```python
from build123d import *

# Parameters (mm, degrees)
F0_W     = 50.8
F0_H     = 50.8
F2_DEPTH = 50.8
F1_R     = 12.7
F3_DEPTH = 51.308
F4_W     = 25.4
F4_H     = 25.4
F5_DEPTH = 12.7
F6_R     = 14.097
F7_DEPTH = 12.7


with BuildPart() as f2:
    # F0 (on Front) → F2 (new body)
    with BuildSketch(Plane.XZ):
        with Locations((-25.4, 25.4)):
            Rectangle(F0_W, F0_H)
    extrude(amount=F2_DEPTH)

    # F1 (on face) → F3 (cut)
    with BuildSketch(Plane.XZ):
        with Locations((-25.4, 25.4)):
            Circle(F1_R)
    extrude(amount=F3_DEPTH, mode=Mode.SUBTRACT)

    # F4 (on face) → F5 (join)
    with BuildSketch(Plane.YZ):
        with Locations((-25.4, 25.4)):
            Rectangle(F4_W, F4_H)
    extrude(amount=F5_DEPTH)

    # F6 (on face) → F7 (join)
    with BuildSketch(Plane(origin=(0, 0, 0), x_dir=(1, 0, 0), z_dir=(0, 0, -1))):
        with Locations((-25.4, 25.4)):
            Circle(F6_R)
    extrude(amount=F7_DEPTH)


solid = f2.part
```
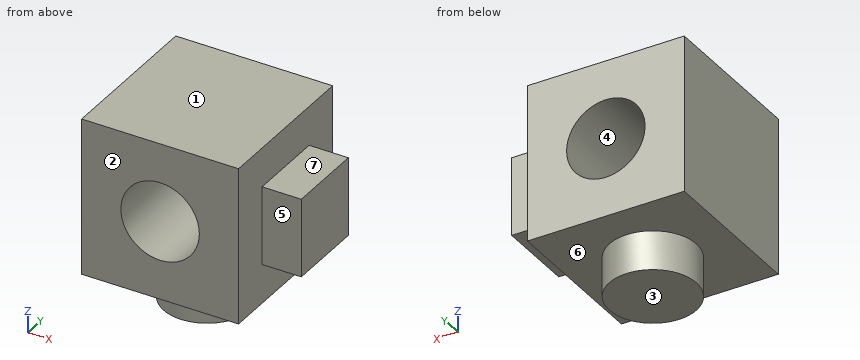
The model under review builds one solid part; all positions refer to its coordinate system, in mm. Face numbers are marked on the shaded views. A direction names the side the tool comes from. Coordinates: 2 decimals unless noted, no trailing zeros. Write each loop counter-clockwise with the first axis right and the second up, starting at its lowest first coordinate (ties: lowest second). Pieces come first, ordered by that corner, then holes. Notation, with made-up numbers: (1.5, 88) - (9.5, 88) arc R19 cw to (9.5, 113) - close; hole circle Ø4 at (46, -27). An arc over 180 degrees is marked (long way). Answer in a Markdown table with one row per item. Add a question column.
Q1. Consider section C-C on x = -25.4. Give the boundary of the cut face in (y, z).
Q2. For the marked faces 5, 6 and 7, list the 3-axis set-ups (+Z, -Z, +X, -X, +Y, -Y) from which the entire face can be reached by the end or side of a thin tool; tool diameter is ignored.
Q3. Draft analysis for pull direction Z (two halves, no side actions). For the marked faces 1, 2, 3 and 4, state which applies: +Z half, -Z half, draft (parallel to the pull), parting line (faces both ways), or undercut.
Q4. Consider section B-B on y = -25.4. Give the boundary of the cut face in (x, z), then the cut area to 3 significant figures.
Q5. Clearance check with flat-ended pins moving along their axes: pin 1 (14 mm diameter, centred on x = 7.5, z = 27.5, fed in from -Y); pin 2 (6.5 mm diameter, centred on x = 9, z = 22.5, fed in from +Y); pin 3 (3 mm diameter, centred on x = -4, y = -18.5, fed in from -Z). State where each tip first meets the part, or that it passes through.
Q6. To check wall thickness, follow line 1 along Z through (x, y) = (-25.4, -23); line 2 along X through (y, z) = (-34, 25); line 3 along X through (y, z) = (-10, 25). State the ranges of each line that lie inside material, in increasing order. Write a range as from..to.
Q7. Consider section D-D on z = 3. Give the boundary of the cut face in (x, y), then the cut area to 3 significant figures.
Q8. Consider section A-A on z = 25.4. Give the boundary of the cut face in (x, y).
Answers below:
| question | item | result |
|---|---|---|
| 1 | outline | (-50.8, 0) - (-39.5, 0) - (-39.5, -12.7) - (-11.3, -12.7) - (-11.3, 0) - (0, 0) - (0, 12.7) - (-50.8, 12.7) - close; (-50.8, 38.1) - (0, 38.1) - (0, 50.8) - (-50.8, 50.8) - close |
| 2 | face 5 | +Z, -Z, +X, -Y |
| 2 | face 6 | -Z |
| 2 | face 7 | +Z, +X, +Y, -Y |
| 3 | face 1 | +Z half |
| 3 | face 2 | draft |
| 3 | face 3 | -Z half |
| 3 | face 4 | undercut |
| 4 | outline | (-50.8, 0) - (-39.5, 0) - (-39.5, -12.7) - (-11.3, -12.7) - (-11.3, 0) - (0, 0) - (0, 12.7) - (12.7, 12.7) - (12.7, 38.1) - (0, 38.1) - (0, 50.8) - (-50.8, 50.8) - close; hole circle Ø25.4 at (-25.4, 25.4) |
| 4 | area | 2,750 mm² |
| 5 | pin 1 | y = -38.1 |
| 5 | pin 2 | y = -12.7 |
| 5 | pin 3 | z = 0 |
| 6 | line 1 | -12.7..12.7, 38.1..50.8 |
| 6 | line 2 | -50.8..-38.09, -12.71..12.7 |
| 6 | line 3 | -50.8..-38.09, -12.71..0 |
| 7 | outline | (-50.8, -50.8) - (0, -50.8) - (0, 0) - (-50.8, 0) - close |
| 7 | area | 2,580 mm² |
| 8 | outline | (-50.8, -50.8) - (-38.1, -50.8) - (-38.1, 0) - (-50.8, 0) - close; (-12.7, -50.8) - (0, -50.8) - (0, -38.1) - (12.7, -38.1) - (12.7, -12.7) - (0, -12.7) - (0, 0) - (-12.7, 0) - close |
